Job drawing, mm, ordinate dimensions from the low corner. One solid piece. A direction names the side the tool comes from. Give positions to 0.01 mm unless a question says otherwise; leave off trailing zeros. Loops run counter-clockwise (first coordinate to the right, second up) from the corner with the lowest first, then second, coordinate; pieces in that order, holes last.
Item 1: Saw through at D-D on x = 19.5. Give the cut face in (y, z), plus the area to 3 significant figures.
Item 2: Probe probe 1 along Y at (x, z) = (25.5, 3.25); probe 2 along X at (y, z) = (7, 10.75); probe 3 along X at (y, z) = (13.25, 1.25). List the from-to ranges inside material, lowest first.
Item 3: Saw through at B-B on y = 14.25. Give the cut face in (x, z), plus the area to 3 significant figures.
Item 4: Mould opens along Y. For the marked faces 4, 5, 6 and 7 say: released by +Y, released by -Y, zero draft, split by the parting line, or undercut.
Item 5: Drop flat-ended pins along their axis: P1, Ø3, axis at y = 3, z = 6, coming from the +X side; P2, Ø2, axis at y = 7.5, z = 1, coming from the +X side; P3, Ø3, axis at y = 10, z = 7, coming from the +X side. Give the stop position or say it passes through.
Item 6: Which spindle directions (+Z, -Z, +X, -X, +Y, -Y) get a long thin tool onto all of the face, cutting with end or side? Do the marked faces 1, 2 and 3. Say none if no direction does.
Item 7: Saw through at C-C on x = 25.25. Give the cut face in (y, z).
Item 8: Saw through at A-A on z = 5.75. Give the cut face in (x, y).
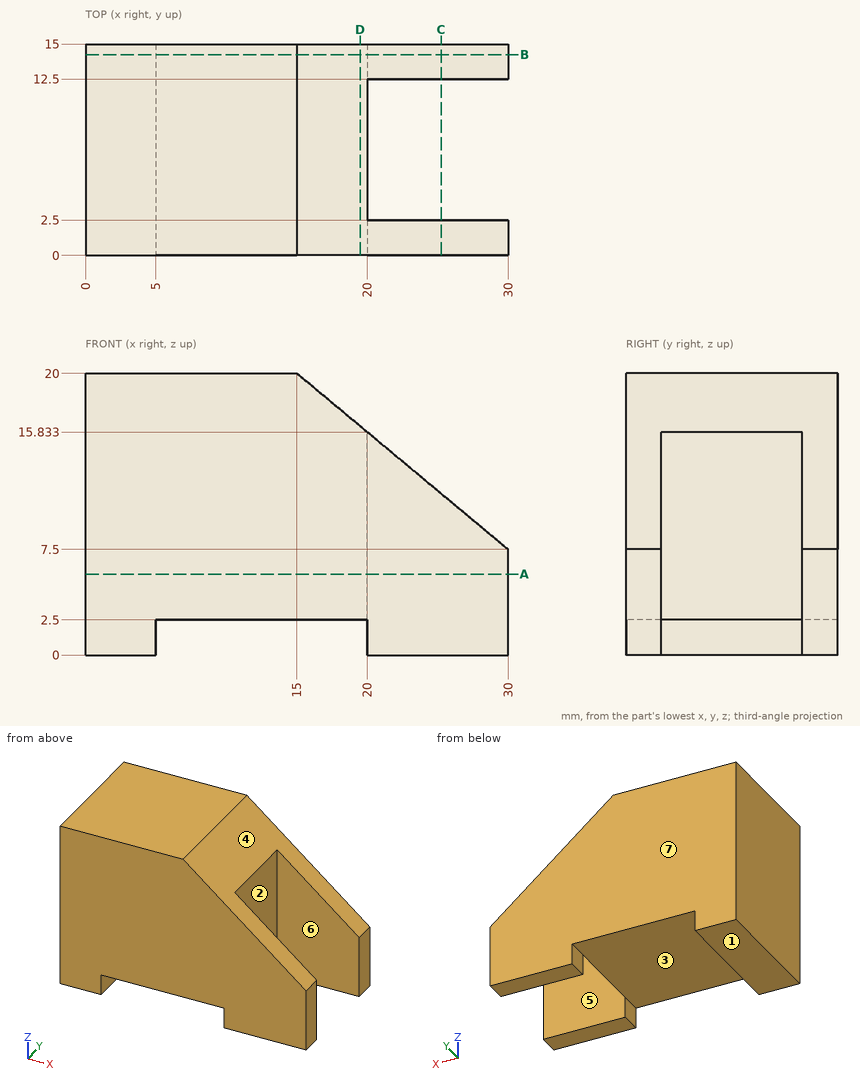
Results below:
1. outline: (0, 2.5) - (15, 2.5) - (15, 16.25) - (0, 16.25) - close
1. area: 206 mm2
2. probe 1: y = 0 to 2.5, 12.5 to 15
2. probe 2: x = 0 to 20
2. probe 3: x = 0 to 5, 20 to 30
3. outline: (0, 0) - (5, 0) - (5, 2.5) - (20, 2.5) - (20, 0) - (30, 0) - (30, 7.5) - (15, 20) - (0, 20) - close
3. area: 469 mm2
4. face 4: zero draft
4. face 5: undercut
4. face 6: undercut
4. face 7: released by +Y
5. P1: stops at x = 30
5. P2: stops at x = 5
5. P3: stops at x = 20
6. face 1: -Z, +X, -X, +Y, -Y
6. face 2: +Z, -Z, +X
6. face 3: -Z, +Y, -Y
7. outline: (0, 0) - (2.5, 0) - (2.5, 11.46) - (0, 11.46) - close; (12.5, 0) - (15, 0) - (15, 11.46) - (12.5, 11.46) - close
8. outline: (0, 0) - (30, 0) - (30, 2.5) - (20, 2.5) - (20, 12.5) - (30, 12.5) - (30, 15) - (0, 15) - close
